Verification items for the finished model (mm, model axes). A direction names the side the tool comes from. Give positions to 0.01 mm unless a question says otherwise; leave off trailing zeros. Write each loop counter-clockwise with the first axis right and the second up, starting at its lowest first coordinate (ties: lowest second). Pieces come first, ordered by that corner, then holes. Notation, with made-up numbers: (-7, -2.75) - (32, -2.75) arc R20 ccw to (32, 10.25) - close; hole circle Ø1 at (84, -18.5). An arc over 180 degrees is marked (long way). Answer as a JSON object with one key per item and string values. Group by question number.
Item 1: Go/stop test with flat-tipped pins: pin 1 (1.5 mm diameter, centred on x = 6.5, y = 40, fed in from +Z); pin 2 (4.5 mm diameter, centred on x = 6.5, y = 5, fed in from -Z); pin 3 (1.8 mm diameter, centred on x = 191.67, y = 37.5, fed in from +Z); pin 4 (17.5 mm diameter, centred on x = 169, y = 20, fed in from +Z). Record where each tip stops, or that it passes through.
Item 2: Scan lines: line 1 along Y through (x, z) = (6.5, 6); line 2 along X through (y, z) = (32, 14.75); line 3 along Y through (x, z) = (141.05, 12.6). Record each from-to range of solid material in increasing order. Write a range as [from, to].
Item 3: Tool access check on faces 5 (the face through (197.19, 39.04, 1.48)), 6 (the face through (183, 9.5, 4)), 7 (the face through (147.05, 22, 11)). Record the directions out of +Z, -Z, +X, -X, +Y, -Y that give a thin tool (end or side, any length) a straight path to the whole face; none if there is none.
Item 4: Draft check along Y on faces 1 (the face through (0, 22, 8)), 2 (the face through (53.545, 23.532, 1.681)), 3 (the face through (102, 45, 8)), 4 (the face through (171, 40, 11)). Enter one of: +Y half, -Y half, draft (parallel to the pull), parting line (faces both ways), or undercut.
Item 5: Sectioned sample at A-A, the plane x = 113. Record the boundary of the cut face in (y, z).
```python
from build123d import *

# Parameters (mm, degrees)
SKETCH_1_W               = 206
SKETCH_1_H               = 45
EXTRUDE_1_DEPTH          = 15
SKETCH_1_4_W             = 85
SKETCH_1_4_H             = 45
CUT_EXTRUDE_1_DEPTH      = 2
SKETCH_1_5_W             = 72.1
SKETCH_1_5_H             = 42
CUT_EXTRUDE_2_DEPTH      = 71
SKETCH_1_6_R             = 3
CUT_EXTRUDE_3_DEPTH      = 42
SKETCH_2_R               = 22
SKETCH_2_R_2             = 4.5
CUT_EXTRUDE_4_DEPTH      = 10
SKETCH_2_3_R             = 4.5
CUT_EXTRUDE_5_DEPTH      = 50
CUT_EXTRUDE_6_DEPTH      = 17
CUT_EXTRUDE_6_DEPTH_BACK = 44
SKETCH_4_R               = 1.5
CUT_EXTRUDE_7_DEPTH      = 14
CHAMFER_1_SIZE           = 1
CHAMFER_2_SIZE           = 2
CUT_EXTRUDE_START        = -10
CUT_EXTRUDE_9_DEPTH      = 11
SKETCH_7_R               = 6
CUT_EXTRUDE_10_DEPTH     = 182
SKETCH_7_4_R             = 8.5
CUT_EXTRUDE_11_DEPTH     = 3
CHAMFER_3_SIZE           = 1
SKETCH_9_R               = 1.25
CUT_EXTRUDE_12_DEPTH     = 182
SKETCH_9_3_R             = 2.5
CUT_EXTRUDE_13_DEPTH     = 3
FILLET_1_R               = 1
SKETCH_10_W              = 47.95
SKETCH_10_H              = 35
CUT_EXTRUDE_14_DEPTH     = 8
SKETCH_11_R              = 1
CUT_EXTRUDE_15_DEPTH     = 3
CHAMFER_4_SIZE           = 1
SKETCH_12_R              = 1
CUT_EXTRUDE_16_DEPTH     = 5


with BuildPart() as part:
    # 草图1 → 凸台-拉伸1 (new body)
    with BuildSketch(Plane.XY):
        with Locations((103, 22.5)):
            Rectangle(SKETCH_1_W, SKETCH_1_H)
    extrude(amount=EXTRUDE_1_DEPTH)

    # 草图1<4> → 切除-拉伸1 (cut)
    with BuildSketch(Plane.XY):
        with Locations((103, 22.5)):
            Rectangle(SKETCH_1_4_W, SKETCH_1_4_H)
    extrude(amount=CUT_EXTRUDE_1_DEPTH, mode=Mode.SUBTRACT)

    # 草图1<5> → 切除-拉伸2 (cut)
    with BuildSketch(Plane.XY):
        with Locations((103, 22.5)):
            Rectangle(SKETCH_1_5_W, SKETCH_1_5_H)
    extrude(amount=CUT_EXTRUDE_2_DEPTH, mode=Mode.SUBTRACT)

    # 草图1<6> → 切除-拉伸3 (cut)
    with BuildSketch(Plane.XY):
        with Locations(Location((63.725, 22.5, 0), (0, 0, 180))):
            Circle(SKETCH_1_6_R)
    extrude(amount=CUT_EXTRUDE_3_DEPTH, mode=Mode.SUBTRACT)

    # 草图2 → 切除-拉伸4 (cut)
    with BuildSketch(Plane(origin=(0, 0, 0), x_dir=(-1, 0, 0), z_dir=(0, 0, -1))):
        with Locations((-31.25, 22.5)):
            Circle(SKETCH_2_R)
        with Locations((-31.25, 22.5)):
            Circle(SKETCH_2_R_2, mode=Mode.SUBTRACT)
    extrude(amount=-CUT_EXTRUDE_4_DEPTH, mode=Mode.SUBTRACT)

    # 草图2<3> → 切除-拉伸5 (cut)
    with BuildSketch(Plane(origin=(0, 0, 0), x_dir=(-1, 0, 0), z_dir=(0, 0, -1))):
        with Locations((-31.25, 22.5)):
            Circle(SKETCH_2_3_R)
    extrude(amount=-CUT_EXTRUDE_5_DEPTH, mode=Mode.SUBTRACT)

    # 草图4 → 切除-拉伸6 (cut, two sides: drawn at the far end of the back side and taken through both)
    with BuildSketch(Plane.XY.offset(15).offset(-CUT_EXTRUDE_6_DEPTH_BACK)):
        with Locations(Location((31.25, 13.5, 0), (0, 0, 180))):
            Circle(SKETCH_4_R)
    extrude(amount=CUT_EXTRUDE_6_DEPTH + CUT_EXTRUDE_6_DEPTH_BACK, mode=Mode.SUBTRACT)

    # 草图5 → 切除-拉伸7 (cut)
    with BuildSketch(Plane(origin=(0, 0, 0), x_dir=(-1, 0, 0), z_dir=(0, 0, -1))):
        with BuildLine():
            Line((-186.665399759, 35.5), (-178.665399759, 35.5))
            ThreePointArc((-178.665399759, 35.5), (-177.165399759, 34), (-178.665399759, 32.5))
            Line((-178.665399759, 32.5), (-186.665399759, 32.5))
            ThreePointArc((-186.665399759, 32.5), (-188.165399759, 34), (-186.665399759, 35.5))
        make_face()
        with BuildLine():
            Line((-186.665399759, 12.5), (-178.665399759, 12.5))
            ThreePointArc((-178.665399759, 12.5), (-177.165399759, 11), (-178.665399759, 9.5))
            Line((-178.665399759, 9.5), (-186.665399759, 9.5))
            ThreePointArc((-186.665399759, 9.5), (-188.165399759, 11), (-186.665399759, 12.5))
        make_face()
        with BuildLine():
            Line((-186.665399759, 24), (-178.665399759, 24))
            ThreePointArc((-178.665399759, 24), (-177.165399759, 22.5), (-178.665399759, 21))
            Line((-178.665399759, 21), (-186.665399759, 21))
            ThreePointArc((-186.665399759, 21), (-188.165399759, 22.5), (-186.665399759, 24))
        make_face()
    extrude(amount=-CUT_EXTRUDE_7_DEPTH, mode=Mode.SUBTRACT)

    # 倒角1
    chamfer_1_edges = [part.edges().sort_by_distance(p)[0] for p in [
        (182.665399759, 21, 0),
        (177.165399759, 22.5, 0),
        (182.665399759, 24, 0),
        (188.165399759, 34, 0),
        (182.665399759, 32.5, 0),
        (177.165399759, 34, 0),
        (182.665399759, 35.5, 0),
        (188.165399759, 11, 0),
        (182.665399759, 9.5, 0),
        (177.165399759, 11, 0),
        (182.665399759, 12.5, 0),
        (188.165399759, 22.5, 0),
    ]]
    chamfer(chamfer_1_edges, length=CHAMFER_1_SIZE)

    # 倒角2
    # the kernel refuses this chamfer: 2 mm, written as the material it takes off along each edge
    with BuildSketch(Plane(origin=(31.25, 22.5, 0), x_dir=(-1, 0, 0), z_dir=(0, -1, 0))) as chamfer_2_piece_1:
        Polygon((22 + CHAMFER_2_SIZE, 0), (22, -CHAMFER_2_SIZE), (22, 0), align=None)
    revolve(axis=Axis((31.25, 22.5, 0), (0, 0, -1)), mode=Mode.SUBTRACT)

    # 切除-拉伸9: read off the stored shape, not the designer's step
    # 切除-拉伸9 outline → 切除-拉伸9 (cut)
    with BuildSketch(Plane(origin=(0, 0, 0), x_dir=(-1, 0, 0), z_dir=(0, 0, -1)).offset(CUT_EXTRUDE_START)):
        with BuildLine():
            ThreePointArc((-25.017060641, 1.401410783), (-31.25, 0.5), (-37.482939359, 1.401410783))
            Line((-37.482939359, 1.401410783), (-39.910254038, 0))
            Line((-39.910254038, 0), (-22.898353456, 0))
            ThreePointArc((-22.898353456, 0), (-22.804826441, 0.034937268), (-22.711445573, 0.070263303))
            Line((-22.711445573, 0.070263303), (-25.017060641, 1.401410783))
        make_face()
        with BuildLine():
            Line((-38.17820323, 45), (-36.296231546, 43.913443142))
            ThreePointArc((-36.296231546, 43.913443142), (-31.25, 44.5), (-26.203768454, 43.913443142))
            Line((-26.203768454, 43.913443142), (-24.32179677, 45))
            Line((-24.32179677, 45), (-38.17820323, 45))
        make_face()
    extrude(amount=CUT_EXTRUDE_9_DEPTH, mode=Mode.SUBTRACT)

    # 草图7 → 切除-拉伸10 (cut)
    with BuildSketch(Plane(origin=(0, 0, 0), x_dir=(-1, 0, 0), z_dir=(0, 0, -1))):
        with Locations((-160.341805483, 22.5)):
            Circle(SKETCH_7_R)
    extrude(amount=-CUT_EXTRUDE_10_DEPTH, mode=Mode.SUBTRACT)

    # 草图7<4> → 切除-拉伸11 (cut)
    with BuildSketch(Plane(origin=(0, 0, 0), x_dir=(-1, 0, 0), z_dir=(0, 0, -1))):
        with Locations((-160.341805483, 22.5)):
            Circle(SKETCH_7_4_R)
    extrude(amount=-CUT_EXTRUDE_11_DEPTH, mode=Mode.SUBTRACT)

    # 倒角3
    chamfer_3_edges = [part.edges().sort_by_distance(p)[0] for p in [
        (168.841805483, 22.5, 0),
    ]]
    chamfer(chamfer_3_edges, length=CHAMFER_3_SIZE)

    # 草图9 → 切除-拉伸12 (cut)
    with BuildSketch(Plane(origin=(0, 0, 0), x_dir=(-1, 0, 0), z_dir=(0, 0, -1))):
        with Locations((-199.5, 40)):
            Circle(SKETCH_9_R)
        with Locations((-199.5, 5)):
            Circle(SKETCH_9_R)
        with Locations((-6.5, 5)):
            Circle(SKETCH_9_R)
        with Locations((-6.5, 40)):
            Circle(SKETCH_9_R)
    extrude(amount=-CUT_EXTRUDE_12_DEPTH, mode=Mode.SUBTRACT)

    # 草图9<3> → 切除-拉伸13 (cut)
    with BuildSketch(Plane(origin=(0, 0, 0), x_dir=(-1, 0, 0), z_dir=(0, 0, -1))):
        with Locations((-199.5, 40)):
            Circle(SKETCH_9_3_R)
        with Locations((-199.5, 5)):
            Circle(SKETCH_9_3_R)
        with Locations((-6.5, 5)):
            Circle(SKETCH_9_3_R)
        with Locations((-6.5, 40)):
            Circle(SKETCH_9_3_R)
    extrude(amount=-CUT_EXTRUDE_13_DEPTH, mode=Mode.SUBTRACT)

    # 圆角1
    fillet_1_edges = [part.edges().sort_by_distance(p)[0] for p in [
        (0, 0, 7.5),
        (206, 0, 7.5),
        (206, 45, 7.5),
        (0, 45, 7.5),
    ]]
    fillet(fillet_1_edges, radius=FILLET_1_R)

    # 草图10 → 切除-拉伸14 (cut)
    with BuildSketch(Plane.XY.offset(15)):
        with Locations((171.025, 22.5)):
            Rectangle(SKETCH_10_W, SKETCH_10_H)
    extrude(amount=-CUT_EXTRUDE_14_DEPTH, mode=Mode.SUBTRACT)

    # 草图11 → 切除-拉伸15 (cut)
    with BuildSketch(Plane.XY.offset(7)):
        with Locations((191.665399759, 37.5)):
            Circle(SKETCH_11_R)
        with Locations((173.665399759, 37.5)):
            Circle(SKETCH_11_R)
        with Locations((173.665399759, 7.5)):
            Circle(SKETCH_11_R)
        with Locations((191.665399759, 7.5)):
            Circle(SKETCH_11_R)
    extrude(amount=-CUT_EXTRUDE_15_DEPTH, mode=Mode.SUBTRACT)

    # 倒角4
    # the kernel refuses this chamfer: 1 mm, written as the material it takes off along each edge
    with BuildSketch(Plane(origin=(142.928317012, 0, 0), x_dir=(0, 1, 0), z_dir=(1, 0, 0)), Plane(origin=(205, 45, 0), x_dir=(0, -1, 0), z_dir=(-1, 0, 0))) as chamfer_4_piece_1:
        Polygon((CHAMFER_4_SIZE, 0), (0, CHAMFER_4_SIZE), (0, 0), align=None)
    extrude(amount=62.071682988, mode=Mode.SUBTRACT)
    with BuildSketch(Plane(origin=(205, 1, 0), x_dir=(0, -1, 0), z_dir=(-1, 0, 0))) as chamfer_4_piece_2:
        Polygon((1 - CHAMFER_4_SIZE, 0), (1, CHAMFER_4_SIZE), (1, 0), align=None)
    revolve(axis=Axis((205, 1, 0), (0, 0, 1)), revolution_arc=90, mode=Mode.SUBTRACT)
    with BuildSketch(Plane(origin=(206, 1, 0), x_dir=(-1, 0, 0), z_dir=(0, 1, 0)), Plane(origin=(0, 44, 0), x_dir=(1, 0, 0), z_dir=(0, -1, 0))) as chamfer_4_piece_3:
        Polygon((CHAMFER_4_SIZE, 0), (0, CHAMFER_4_SIZE), (0, 0), align=None)
    extrude(amount=43, mode=Mode.SUBTRACT)
    with BuildSketch(Plane(origin=(205, 44, 0), x_dir=(0, 1, 0), z_dir=(-1, 0, 0))) as chamfer_4_piece_4:
        Polygon((1 - CHAMFER_4_SIZE, 0), (1, -CHAMFER_4_SIZE), (1, 0), align=None)
    revolve(axis=Axis((205, 44, 0), (0, 0, -1)), revolution_arc=90, mode=Mode.SUBTRACT)
    with BuildSketch(Plane(origin=(37.33857105, 0, 0), x_dir=(0, 0, 1), z_dir=(1, 0, 0))) as chamfer_4_piece_5:
        Polygon((CHAMFER_4_SIZE, 0), (0, -CHAMFER_4_SIZE), (0, 0), align=None)
    extrude(amount=25.733111938, mode=Mode.SUBTRACT)
    with BuildSketch(Plane(origin=(63.071682988, 45, 0), x_dir=(0, 0, 1), z_dir=(-1, 0, 0))) as chamfer_4_piece_6:
        Polygon((CHAMFER_4_SIZE, 0), (0, -CHAMFER_4_SIZE), (0, 0), align=None)
    extrude(amount=27.841897523, mode=Mode.SUBTRACT)
    with BuildSketch(Plane(origin=(1, 0, 0), x_dir=(0, 0, 1), z_dir=(1, 0, 0))) as chamfer_4_piece_7:
        Polygon((CHAMFER_4_SIZE, 0), (0, -CHAMFER_4_SIZE), (0, 0), align=None)
    extrude(amount=24.470036444, mode=Mode.SUBTRACT)
    with BuildSketch(Plane(origin=(27.270214535, 45, 0), x_dir=(0, 0, 1), z_dir=(-1, 0, 0))) as chamfer_4_piece_8:
        Polygon((CHAMFER_4_SIZE, 0), (0, -CHAMFER_4_SIZE), (0, 0), align=None)
    extrude(amount=26.270214535, mode=Mode.SUBTRACT)
    with BuildSketch(Plane(origin=(1, 1, 0), x_dir=(0, -1, 0), z_dir=(1, 0, 0))) as chamfer_4_piece_9:
        Polygon((1 - CHAMFER_4_SIZE, 0), (1, -CHAMFER_4_SIZE), (1, 0), align=None)
    revolve(axis=Axis((1, 1, 0), (0, 0, -1)), revolution_arc=90, mode=Mode.SUBTRACT)
    with BuildSketch(Plane(origin=(1, 44, 0), x_dir=(0, 1, 0), z_dir=(1, 0, 0))) as chamfer_4_piece_10:
        Polygon((1 - CHAMFER_4_SIZE, 0), (1, CHAMFER_4_SIZE), (1, 0), align=None)
    revolve(axis=Axis((1, 44, 0), (0, 0, 1)), revolution_arc=90, mode=Mode.SUBTRACT)

    # 草图12 → 切除-拉伸16 (cut)
    with BuildSketch(Plane.XY.offset(15)):
        with Locations((61.95, 40.5)):
            Circle(SKETCH_12_R)
        with Locations((61.95, 4.5)):
            Circle(SKETCH_12_R)
        with Locations((141.05, 4.5)):
            Circle(SKETCH_12_R)
        with Locations((141.05, 40.5)):
            Circle(SKETCH_12_R)
    extrude(amount=-CUT_EXTRUDE_16_DEPTH, mode=Mode.SUBTRACT)


solid = part.part
```
Geometry check:
{
 "1": {"pin 1": "through", "pin 2": "z = 3", "pin 3": "z = 4", "pin 4": "z = 7"},
 "2": {"line 1": "[0, 3.75], [6.25, 38.75], [41.25, 45]", "line 2": "[0, 66.95], [139.05, 147.05], [195, 206]", "line 3": "[0, 3.5], [5.5, 39.5], [41.5, 45]"},
 "3": {"face 5": "-Z", "face 6": "+Z, -Z", "face 7": "+Z"},
 "4": {"face 1": "draft", "face 2": "undercut", "face 3": "+Y half", "face 4": "undercut"},
 "5": {"outline": "(0, 2) - (1.5, 2) - (1.5, 15) - (0, 15) - close; (43.5, 2) - (45, 2) - (45, 15) - (43.5, 15) - close"}
}
